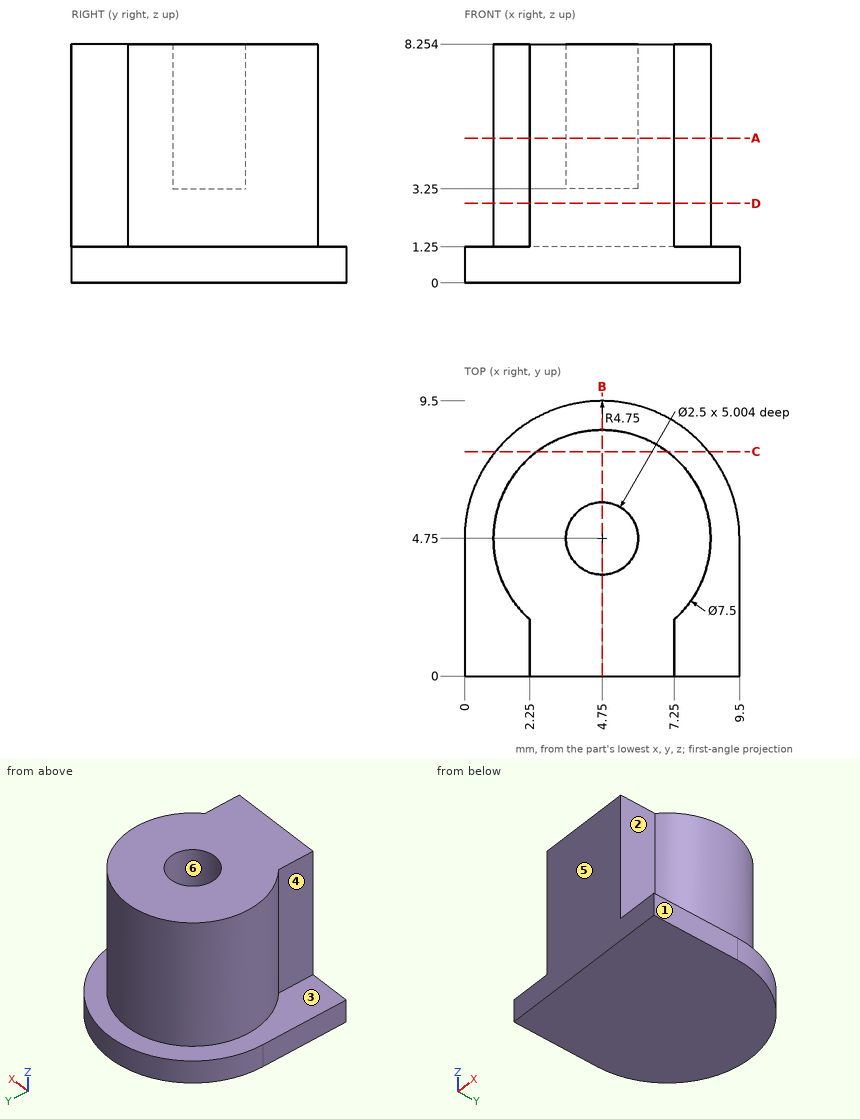
Input: dimensioned drawing with shaded views. Units: mm. Origin: part minimum x, y, z. A direction names the side the tool comes from. Give positions to 0.01 mm unless a question says otherwise; leave off trailing zeros. Write each loop counter-clockwise with the first axis right and the second up, starting at its lowest first coordinate (ties: lowest second). Pieces come first, ordered by that corner, then holes.
Q1. Section C-C, the plane y = 7.75. Output: boundary loops of the cut face in (x, z).
Q2. Material intervals for probe 1 along Y at (x, z) = (4.75, 5); probe 2 along X at (y, z) = (4.75, 5.55); probe 3 along Z at (x, y) = (9.25, 4), sorted ascending.
Q3. First-contact query: P1, Ø0.8, axis at x = 5, y = 5, coming from the +Z side; P2, Ø1.6, axis at y = 1, z = 5.5, coming from the +X side; P3, Ø1.5, axis at x = 4, y = 5.5, coming from the -Z side; P4, Ø1, axis at y = 1, z = 5.5, coming from the -X side. Flat tips, straight axial feed; report the tip coordinate or a pass-through.
Q4. Section A-A, the plane z = 5. Output: boundary loops of the cut face in (x, y).
Q5. Pull-direction query (Y, two-part tool) for the marked faces 4, 5 and 6; classes: pulls with the +Y half, pulls with the -Y half, needs draft (parallel to the pull), parting line crosses it, or undercut.
Q6. Section D-D, the plane z = 2.75. Output: boundary loops of the cut face in (x, y).
Q7. Set-up query: the marked faces 1, 2 and 3. Return all of +Z, -Z, +X, -X, +Y, -Y with unobstructed straight access to the full face (end or side cutting, diameter ignored); none if empty.
Q8. Section B-B, the plane x = 4.75. Output: boundary loops of the cut face in (y, z), plus the area to 3 significant figures.
Filled in:
1. outline: (1.07, 0) - (8.43, 0) - (8.43, 1.25) - (7, 1.25) - (7, 8.25) - (2.5, 8.25) - (2.5, 1.25) - (1.07, 1.25) - close
2. probe 1: y = 0 to 3.5, 6 to 8.5
2. probe 2: x = 1 to 3.5, 6 to 8.5
2. probe 3: z = 0 to 1.25
3. P1: stops at z = 3.25
3. P2: stops at x = 7.25
3. P3: stops at z = 0
3. P4: stops at x = 2.25
4. outline: (2.25, 0) - (7.25, 0) - (7.25, 1.95) arc R3.75 ccw (long way) to (2.25, 1.95) - close; hole circle Ø2.5 at (4.75, 4.75)
5. face 4: needs draft
5. face 5: pulls with the -Y half
5. face 6: undercut
6. outline: (2.25, 0) - (7.25, 0) - (7.25, 1.95) arc R3.75 ccw (long way) to (2.25, 1.95) - close
7. face 1: +Z, -Z, +X, +Y, -Y
7. face 2: +Z, +X, -Y
7. face 3: +Z
8. outline: (0, 0) - (9.5, 0) - (9.5, 1.25) - (8.5, 1.25) - (8.5, 8.25) - (6, 8.25) - (6, 3.25) - (3.5, 3.25) - (3.5, 8.25) - (0, 8.25) - close
8. area: 58.9 mm2
